Can you work these out from the model? Positions are in its coordinate system, mm. Face numbers are marked on the shaded views. A direction names the side the tool comes from. Coordinates: 2 decimals unless noted, no trailing zeros. Order: outer loops, then holes, each group sorted by start corner. A loop starts at its lowest first (then second) coordinate and runs counter-clockwise, first axis right, second up. Notation, with made-up numbers: (-2, -21.75) -> (34, -21.75) arc R34 cw to (34, 16.25) -> close; hole circle Ø5 at (27, 75.5). An arc over 180 degrees is marked (long way). Write item = value, one per line. Start each with the question number.
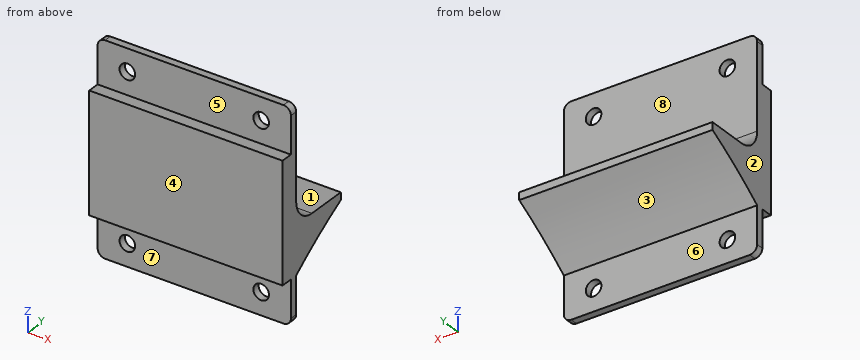
Autodesk Inventor part; units mm, degrees
ref_plane "YZ Plane" through (0, 0, 0) normal (1, 0, 0) x (0, 1, 0)
ref_plane "XZ Plane" through (0, 0, 0) normal (0, 1, 0) x (-1, 0, 0)
ref_plane "XY Plane" through (0, 0, 0) normal (0, 0, 1) x (1, 0, 0)
sketch "Эскиз1" plane through (0, 0, 0) normal (0, 1, 0) x (-1, 0, 0)
  line L0 (0, 0) -> (52, 0)
  line L1 (52, 0) -> (52, -56)
  line L2 (52, -56) -> (0, -56)
  line L3 (0, -56) -> (0, 0)
  dimension "d0" = 56
  dimension "d9" = 52
extrude "Выдавливание1" add sketch "Эскиз1" along normal blind 5.2
sketch "Эскиз2" plane through (0, 0, 0) normal (1, 0, 0) x (0, 0, -1)
  line L0 (56, 0) -> (0, 0)
  line L1 (0, 0) -> (12, 0)
  line L2 (12, 0) -> (12, 3.2)
  line L3 (12, 3.2) -> (0, 3.2)
  line L4 (0, 3.2) -> (0, 0)
  line L5 (56, 0) -> (56, 5.2)
  line L6 (56, 0) -> (44, 0)
  line L7 (44, 0) -> (44, 3.2)
  line L8 (44, 3.2) -> (56, 3.2)
  line L9 (56, 3.2) -> (56, 0)
  dimension "d3" = 12
  dimension "d4" = 3.2
  dimension "d5" = 12
  dimension "d6" = 3.2
extrude "Выдавливание2" cut sketch "Эскиз2" against normal up to surface (52 mm away)
sketch "Эскиз3" plane through (0, 3.2, -12) normal (0, -1, 0) x (1, 0, 0)
  circle A0 centre (-8, 6) radius 2.1
  line L0 (0, 12) -> (0, 0)
  line L1 (-52, 12) -> (0, 12)
  circle A1 centre (-44, 6) radius 2.1
  line L2 (-52, 0) -> (-52, 12)
  circle A2 centre (-44, -38) radius 2.1
  line L3 (-52, -44) -> (-52, -32)
  line L4 (0, -44) -> (-52, -44)
  circle A3 centre (-8, -38) radius 2.1
  line L5 (0, -32) -> (0, -44)
  point P0 (0, 6)
  dimension "d10" = 4.2
  dimension "d11" = 8
  dimension "d12" = 6
  dimension "d13" = 4.2
  dimension "d14" = 6
  dimension "d15" = 8
  dimension "d16" = 4.2
  dimension "d17" = 8
  dimension "d18" = 6
  dimension "d19" = 4.2
  dimension "d20" = 8
  dimension "d21" = 6
extrude "Выдавливание3" cut sketch "Эскиз3" against normal blind 10
fillet "Сопряжение1" radius 2 4 edges at (0, 4.2, 0) (0, 4.2, -56) (-52, 4.2, -56) (-52, 4.2, 0)
sketch "Эскиз4" plane through (0, 0, -12) normal (1, 0, 0) x (0, 0, -1)
  line L0 (31.9749, 5.2) -> (18.9749, 5.2)
  line L1 (18.9749, 22.2) -> (18.9749, 5.2)
  line L2 (18.9749, 22.2) -> (20.9749, 22.2)
  arc A0 (20.9749, 22.2) -> (31.9749, 5.2) centre (135.2876, 84.1082) ccw
  point P0 (-12, 0)
  dimension "d26" = 13
  dimension "d34" = 2
  dimension "d35" = 130
extrude "Выдавливание4" add sketch "Эскиз4" against normal up to surface (52 mm away)
fillet "Сопряжение3" radius 6 1 edges at (-26, 5.2, -30.9749)
(1) For the marked faces 4, 5, 6, 7 and 8, which set-ups out of +Z, -Z, +X, -X, +Y, -Y let a thin tool reach every point of the face, with its end or its side?
(2) Thinking about a two-plate mould opening in Z: for the marked faces 1, 2 and 3, which applies, +Z half, -Z half, draft (parallel to the pull), parting line (faces both ways), or undercut?
(3) Imagine slicing it at C-C (z = -46.5). Write out the boundary of the cut face in (x, y), plus the area to 3 significant figures.
(4) Imagine slicing it at B-B (x = -44). Write out the boundary of the cut face in (y, z), plus the area to 3 significant figures.
(5) For P1, Ø6.5, axis at x = -44, z = -6, coming from the +Y side; P2, Ø6, axis at x = -34.5, y = 9, coming from the -Z side; P3, Ø2.5, axis at x = -19, y = 1.5, coming from the -Z side; P4, Ø3.5, axis at x = -44, z = -50, coming from the -Y side, each with a flat end and sliding along its axis, tell me the tip position at first contact or that it passes through.
(6) Imagine slicing it at D-D (y = 6.25). Write out the boundary of the cut face in (x, z).
(7) Imagine slicing it at A-A (z = -6). Write out the boundary of the cut face in (x, y), plus the area to 3 significant figures.
(8) If I drill on L1, parallel to Z at x = -44, y = 4.2; L2, parallel to Y at x = -6.5, z = -44.5; L3, parallel to Y at x = -11, z = -23, over which ranges is the centre line in solid material (lowest first)? Write a range as from..to.
Result set:
q1.face_4 = +Z, -Z, +X, -X, -Y
q1.face_5 = +Z, +X, -X, -Y
q1.face_6 = -Z, +X, -X, +Y
q1.face_7 = -Z, +X, -X, -Y
q1.face_8 = +Z, +X, -X, +Y
q2.face_1 = +Z half
q2.face_2 = draft
q2.face_3 = -Z half
q3.outline = (-52, 3.2) -> (0, 3.2) -> (0, 5.2) -> (-52, 5.2) -> close
q3.area = 104 mm2
q4.outline = (0, -44) -> (3.2, -44) -> (3.2, -47.9) -> (5.2, -47.9) -> (5.2, -43.97) arc R130 cw to (22.2, -32.97) -> (22.2, -30.97) -> (11.2, -30.97) arc R6 cw to (5.2, -24.97) -> (5.2, -8.1) -> (3.2, -8.1) -> (3.2, -12) -> (0, -12) -> close; (3.2, -56) -> (5.2, -56) -> (5.2, -52.1) -> (3.2, -52.1) -> close; (3.2, -3.9) -> (5.2, -3.9) -> (5.2, 0) -> (3.2, 0) -> close
q4.area = 327 mm2
q5.P1 = 5.2
q5.P2 = -43.37
q5.P3 = -44
q5.P4 = through
q6.outline = (-52, -43.18) -> (0, -43.18) -> (0, -28.37) -> (-52, -28.37) -> close
q7.outline = (-52, 3.2) -> (-46.1, 3.2) -> (-46.1, 5.2) -> (-52, 5.2) -> close; (-41.9, 3.2) -> (-10.1, 3.2) -> (-10.1, 5.2) -> (-41.9, 5.2) -> close; (-5.9, 3.2) -> (0, 3.2) -> (0, 5.2) -> (-5.9, 5.2) -> close
q7.area = 87.2 mm2
q8.L1 = -56..-52.1, -47.9..-8.1, -3.9..0
q8.L2 = 3.2..5.2
q8.L3 = 0..5.2
